Geometry check sheet. Reference: the model listing, model coordinates, mm. A direction names the side the tool comes from. Round coordinates to 2 decimals unless told otherwise and drop trailing zeros. Order: outer loops, then holes, each group sorted by start corner. A loop starts at its lowest first (then second) coordinate and runs counter-clockwise, first axis right, second up. Notation, with made-up numbers: (-15.75, 68) - (7.25, 68) arc R26 cw to (7.25, 89) - close; hole circle Ø1 at (87.25, -18). An arc over 180 degrees is marked (long way). Answer as CSV lines item,"result". Start each with the question number.
Autodesk Inventor part; units mm, degrees
ref_plane "YZ Plane" through (0, 0, 0) normal (1, 0, 0) x (0, 1, 0)
ref_plane "XZ Plane" through (0, 0, 0) normal (0, 1, 0) x (-1, 0, 0)
ref_plane "XY Plane" through (0, 0, 0) normal (0, 0, 1) x (1, 0, 0)
sketch "スケッチ1" plane through (0, 0, 0) normal (0, 0, 1) x (1, 0, 0)
  line L0 (0, 0) -> (15, 0)
  line L1 (15, 0) -> (15, 15)
  line L2 (15, 15) -> (0, 15)
  line L3 (0, 15) -> (0, 0)
  dimension "d0" = 15
  dimension "d1" = 15
extrude "押し出し1" add sketch "スケッチ1" along normal blind 140
sketch "スケッチ3" plane through (0, 0, 0) normal (0, 0, -1) x (-1, 0, 0)
  line L0 (0, 0) -> (-15, 0)
  line L1 (-15, 0) -> (-15, 15)
  line L2 (-15, 15) -> (0, 15)
  line L3 (0, 15) -> (0, 0)
  dimension "d18" = 15
  dimension "d19" = 15
extrude "押し出し2" add sketch "スケッチ3" along normal blind 200
sketch "スケッチ4" plane through (0, 0, -200) normal (0, 0, -1) x (-1, 0, 0)
  point P0 (0, 0)
sketch "スケッチ6" plane through (0, 0, 140) normal (0, 0, 1) x (1, 0, 0)
  line L0 (0, 0) -> (0, 15)
  line L1 (15, 15) -> (15, 0)
  line L2 (0, 0) -> (15, 0)
  line L3 (15, 0) -> (15, 15)
  line L4 (15, 15) -> (0, 15)
  line L5 (0, 15) -> (0, 0)
extrude "押し出し3" cut sketch "スケッチ6" against normal blind 15
sketch "スケッチ7" plane through (0, 0, 125) normal (0, 0, 1) x (1, 0, 0)
  point P0 (0, 0)
  point P1 (0, 0)
sketch "スケッチ8" plane through (0, 0, -200) normal (-1, 0, 0) x (0, 0, 1)
  circle A0 centre (240, 7.5) radius 1.6
  line L0 (0, 15) -> (325, 15)
  line L1 (325, 0) -> (325, 15)
  point P0 (200, 0)
  dimension "d34" = 3.2
  dimension "d35" = 7.5
  dimension "d36" = 85
hole "穴3" at (0, 7.5, 40) direction (1, 0, 0) diameter 3.2 end through all
sketch "スケッチ9" plane through (0, 0, -200) normal (-1, 0, 0) x (0, 0, 1)
  circle A0 centre (250, 7.5) radius 1.6
  line L0 (0, 0) -> (325, 0)
  line L1 (325, 0) -> (325, 15)
  circle A1 centre (230, 7.5) radius 1.6
  point P0 (200, 0)
  dimension "d44" = 3.2
  dimension "d45" = 7.5
  dimension "d46" = 75
  dimension "d47" = 3.2
  dimension "d48" = 7.5
  dimension "d49" = 20
hole "穴4" at (0, 7.5, 30) at (0, 7.5, 50) direction (1, 0, 0) diameter 3.2 end through all
sketch "スケッチ10" plane through (0, 15, -200) normal (0, 1, 0) x (1, 0, 0)
  circle A0 centre (7.5, -318) radius 1.6
  line L0 (0, 0) -> (0, -325)
  line L1 (0, -325) -> (15, -325)
  circle A1 centre (7.5, -311) radius 1.6
  circle A2 centre (7.5, -304) radius 1.6
  point P0 (0, -200)
  dimension "d57" = 3.2
  dimension "d58" = 7.5
  dimension "d59" = 7
  dimension "d60" = 3.2
  dimension "d61" = 3.2
  dimension "d62" = 7
  dimension "d63" = 7
hole "穴5" at (7.5, 15, 104) at (7.5, 15, 111) at (7.5, 15, 118) direction (0, -1, 0) diameter 3.2 end through all
sketch "スケッチ11" plane through (15, 0, -200) normal (1, 0, 0) x (0, 0, -1)
  line L0 (0, 15) -> (0, 0)
  line L1 (-325, 0) -> (0, 0)
  point P0 (-200, 0)
  point P1 (-30, 7.5)
  point P2 (-40, 7.5)
  point P3 (-50, 7.5)
  dimension "d71" = 30
  dimension "d72" = 7.5
  dimension "d73" = 10
  dimension "d74" = 10
hole "穴6" at (15, 7.5, -150) at (15, 7.5, -160) at (15, 7.5, -170) direction (-1, 0, 0) diameter 3.2 end through all
sketch "スケッチ12" plane through (0, 0, 125) normal (0, 0, 1) x (1, 0, 0)
  line L0 (1.5, 13.5) -> (13.5, 13.5)
  line L1 (13.5, 13.5) -> (13.5, 1.5)
  line L2 (13.5, 1.5) -> (1.5, 1.5)
  line L3 (1.5, 1.5) -> (1.5, 13.5)
  line L4 (0, 15) -> (15, 15)
  line L5 (0, 0) -> (0, 15)
  dimension "d82" = 12
  dimension "d83" = 12
  dimension "d84" = 1.5
  dimension "d85" = 1.5
extrude "押し出し4" cut sketch "スケッチ12" against normal blind 450
sketch "スケッチ13" plane through (0, 15, -200) normal (0, 1, 0) x (1, 0, 0)
  point P0 (0, -200)
properties part number "射出_角柱5" material "アルミニウム 6061"
1. Section check A-A on z = 74.5. Record the boundary of the cut face in (x, y), plus the area to 3 significant figures.
2. Go/stop test with a flat-tipped pin: pin 1 Ø2.5 at (y, z) = (7.5, 30) entering from -X. Record where the tip stops, or that it passes through.
3. Access from +Z, -Z, +X, -X, +Y, -Y to the whole of each face (thin tool, end or side, straight path). Record for faces 5 (the face through (8, 15, -40)), 6 (the face through (8, 1.5, -35)).
4. Draft check along X on faces 1 (the face through (1, 8, -200)), 2 (the face through (15, 7, -40)), 3 (the face through (0, 8, -40)), 4 (the face through (7, 13.5, -35)). Enter one of: released by +X, released by -X, zero draft, split by the parting line, or undercut.
5. Thickness scan on probe 1 along Z at (x, y) = (7.5, 14.45); probe 2 along X at (y, z) = (3, 96.5). Record the ranges inside material, lowest first.
Numbers:
1,outline,"(0, 0) - (15, 0) - (15, 15) - (0, 15) - close; hole (1.5, 1.5) - (13.5, 1.5) - (13.5, 13.5) - (1.5, 13.5) - close"
1,area,"81.0 mm2"
2,pin 1,"passes through"
3,face 5,"+Z, -Z, +X, -X, +Y"
3,face 6,"+Z, -Z"
4,face 1,"zero draft"
4,face 2,"released by +X"
4,face 3,"released by -X"
4,face 4,"undercut"
5,probe 1,"z = -200 to 102.4, 105.6 to 109.4, 112.6 to 116.4, 119.6 to 125"
5,probe 2,"x = 0 to 1.5, 13.5 to 15"
